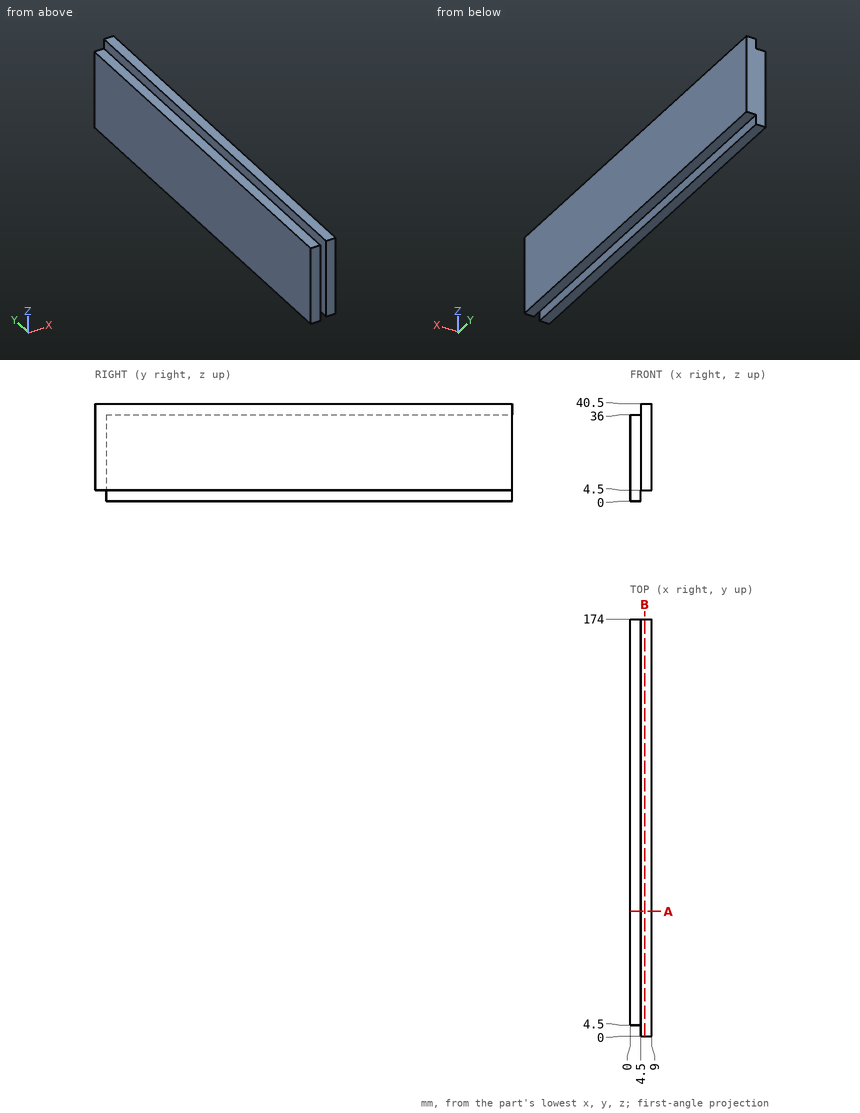
Input: dimensioned drawing with shaded views. Units: mm. Origin: part minimum x, y, z. Coordinates: 2 decimals unless noted, no trailing zeros. Loops run counter-clockwise (first coordinate to the right, second up) from the corner with the lowest first, then second, coordinate; pieces in that order, holes last. Notation, with made-up numbers: (31.5, 37) -> (85.5, 37) arc R17 cw to (85.5, 51) -> close; hole circle Ø11 at (59, 45). An arc over 180 degrees is marked (long way). One line per item, written item: value. Start each with the question number.
Q1. Section query A-A, the plane y = 52. Return the cut outline in (x, z), and give its area (3 significant figures).
Q2. Section query B-B, the plane x = 6. Return the cut outline in (y, z), and give its area (3 significant figures).
Q3. Contact query for flat-ended pins moving along their axis: P1, Ø2, axis at y = 53.5, z = 2.5, coming from the +X side; P2, Ø1.3, axis at x = 6, y = 97.5, coming from the -Z side; P3, Ø1.3, axis at x = 2, y = 106.5, coming from the +Z side. Output: stop coordinate, or through.
Q4. Line query: line 1 along Z through (x, y) = (3.5, 11); line 2 along Y through (x, z) = (2, 34); line 3 along Z through (x, y) = (8.5, 20). Output: solid intervals per line, ascending.
Results:
1. outline: (0, 0) -> (4.5, 0) -> (4.5, 4.5) -> (9, 4.5) -> (9, 40.5) -> (4.5, 40.5) -> (4.5, 36) -> (0, 36) -> close
1. area: 324 mm^2
2. outline: (0, 4.5) -> (174, 4.5) -> (174, 40.5) -> (0, 40.5) -> close
2. area: 6,260 mm^2
3. P1: x = 4.5
3. P2: z = 4.5
3. P3: z = 36
4. line 1: 0 to 36
4. line 2: 4.5 to 174
4. line 3: 4.5 to 40.5
